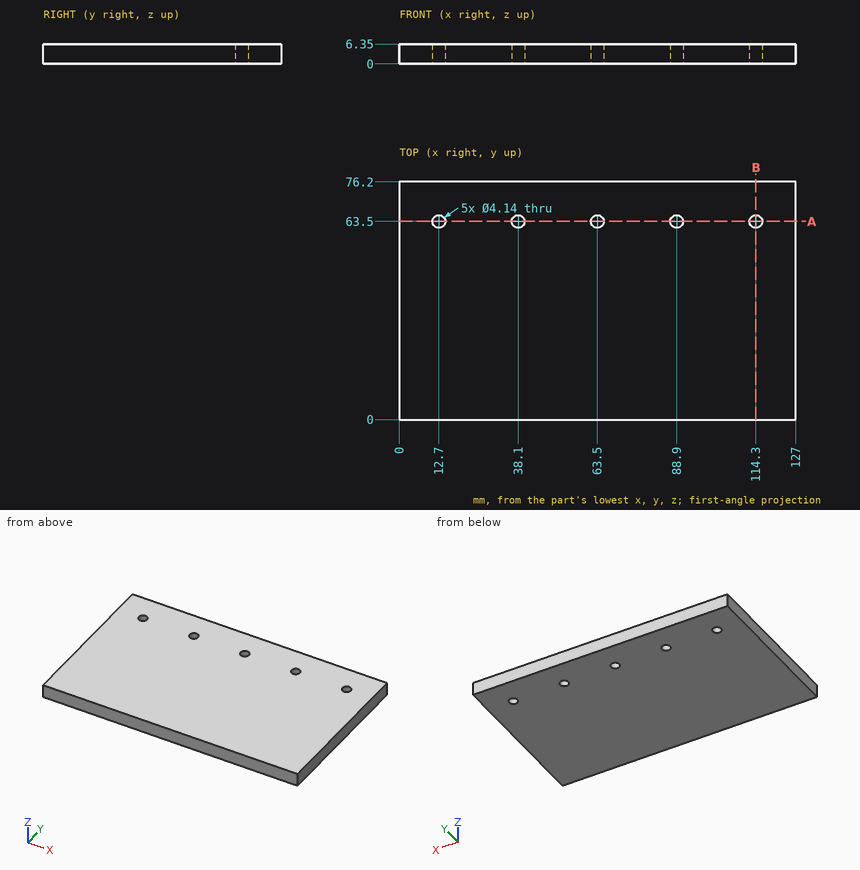
For this review, use the dimensioned drawing (mm, ordinates from the lowest corner) and the shaded views. Round coordinates to 2 decimals unless told otherwise and drop trailing zeros. Order: outer loops, then holes, each group sorted by start corner. A loop starts at its lowest first (then second) coordinate and runs counter-clockwise, first axis right, second up.
1) For L1, parallel to X at y = 63.5, z = 3, list the stretches that pass through material, from the lowest coordinate up.
The answers:
L1: x = 0 to 10.63, 14.77 to 36.03, 40.17 to 61.43, 65.57 to 86.83, 90.97 to 112.23, 116.37 to 127
2) Consider section B-B (x = 114.3). State the section outline as (y, z) points, plus the area to 3 significant figures.
The answers:
outline: (0, 0) - (61.43, 0) - (61.43, 6.35) - (0, 6.35) - close; (65.57, 0) - (76.2, 0) - (76.2, 6.35) - (65.57, 6.35) - close
area: 458 mm2
3) Consider section A-A (y = 63.5). State the section outline as (x, z) points, plus the area to 3 significant figures.
The answers:
outline: (0, 0) - (10.63, 0) - (10.63, 6.35) - (0, 6.35) - close; (14.77, 0) - (36.03, 0) - (36.03, 6.35) - (14.77, 6.35) - close; (40.17, 0) - (61.43, 0) - (61.43, 6.35) - (40.17, 6.35) - close; (65.57, 0) - (86.83, 0) - (86.83, 6.35) - (65.57, 6.35) - close; (90.97, 0) - (112.23, 0) - (112.23, 6.35) - (90.97, 6.35) - close; (116.37, 0) - (127, 0) - (127, 6.35) - (116.37, 6.35) - close
area: 675 mm2
